Geometry: final body of the model. Coordinates: model frame, mm. Round coordinates to 2 decimals unless told otherwise and drop trailing zeros. Loops run counter-clockwise (first coordinate to the right, second up) from the corner with the lowest first, then second, coordinate; pieces in that order, holes last. Notation, with made-up numbers: (34, -17.75) - (93, -17.75) arc R25 ccw to (93, 1.25) - close; hole circle Ø4 at (12.5, -8). An arc over 180 degrees is marked (long way). Write item = value, one per line. Start each with the question number.
Item 1: Section D-D (y = 2.45). Count the separate pieces of the cut face and the enclosed holes in it, plus the area to 3 significant figures.
Item 2: Section C-C (x = -19). Return loops of the section in (y, z).
Item 3: Section A-A (x = 22). Return loops of the section in (y, z) (3 decimals), plus the area to 3 significant figures.
Item 4: Section B-B (z = -28). Return loops of the section in (x, y).
Item 5: Line query: line 1 (X direction, y = 1.5, z = -17.5); line 2 (Z direction, x = -22.5, y = 2.1); line 3 (X direction, y = 2.3, z = -9.5). Output: solid intervals per line, ascending. Write a range as from..to.
Item 6: First-contact query: pin 1 (1 mm diameter, centred on y = 1, z = -23.5, fed in from +X); pin 2 (2.5 mm diameter, centred on y = 2, z = -17.5, fed in from -X); pin 3 (2.5 mm diameter, centred on y = 2, z = -57.5, fed in from +X). Flat tips, straight axial feed; report the tip coordinate or a pass-through.
from build123d import *

# Parameters (mm, degrees)
SKETCH1_R           = 1.5875
SKETCH1_R_2         = 2.0955
SKETCH1_W           = 7.0612
SKETCH1_H           = 27.94
BOSS_EXTRUDE1_DEPTH = 4.699
FILLET1_R           = 2.54


with BuildPart() as part:
    # Sketch1 → Boss-Extrude1 (new body)
    with BuildSketch(Plane(origin=(0, 0, 0), x_dir=(1, 0, 0), z_dir=(0, 1, 0))):
        Polygon((0, 0), (30.48, 0), (30.48, 29.845), (32.385, 31.75), (32.385, 50.546), (-3.048, 50.546), (-3.048, 61.722), (-30.48, 61.722), (-30.48, 49.5427), (-35.2425, 44.7802), (-35.2425, 36.5252), (-30.48, 31.7627), (-30.48, 0), align=None)
        with Locations(Location((-0.9906, 40.6527, 0), (0, 0, 270))):
            Circle(SKETCH1_R, mode=Mode.SUBTRACT)
        with Locations(Location((-12.55014, 55.50916, 0), (0, 0, 270))):
            Circle(SKETCH1_R_2, mode=Mode.SUBTRACT)
        with Locations(Location((-22.40026, 55.50916, 0), (0, 0, 270))):
            Circle(SKETCH1_R_2, mode=Mode.SUBTRACT)
        with Locations(Location((-12.55014, 6.08584, 0), (0, 0, 270))):
            Circle(SKETCH1_R_2, mode=Mode.SUBTRACT)
        with Locations(Location((-22.40026, 6.08584, 0), (0, 0, 270))):
            Circle(SKETCH1_R_2, mode=Mode.SUBTRACT)
        Polygon((5.461, 5.715), (25.781, 5.715), (25.781, 38.0492), (28.575, 38.0492), (28.575, 46.736), (5.461, 46.736), (5.461, 43.2562), (2.5273, 43.2562), (2.5273, 38.0492), (5.461, 38.0492), align=None, mode=Mode.SUBTRACT)
        Polygon((-27.5082, 10.668), (-7.4422, 10.668), (-7.4422, 38.0492), (-4.5085, 38.0492), (-4.5085, 43.2562), (-7.4422, 43.2562), (-7.4422, 50.927), (-27.5082, 50.927), (-27.5082, 43.2562), (-32.5755, 43.2562), (-32.5755, 38.0492), (-27.5082, 38.0492), align=None, mode=Mode.SUBTRACT)
        with Locations((-0.9906, 20.32)):
            Rectangle(SKETCH1_W, SKETCH1_H, mode=Mode.SUBTRACT)
    extrude(amount=BOSS_EXTRUDE1_DEPTH)

    # Fillet1
    fillet1_edges = [part.edges().sort_by_distance(p)[0] for p in [
        (-3.048, 2.3495, -50.546),
        (32.385, 2.3495, -50.546),
        (32.385, 2.3495, -31.75),
        (30.48, 2.3495, -29.845),
        (30.48, 2.3495, 0),
        (-30.48, 2.3495, 0),
        (-30.48, 2.3495, -31.7627),
        (-35.2425, 2.3495, -36.5252),
        (-35.2425, 2.3495, -44.7802),
        (-30.48, 2.3495, -49.5427),
        (-30.48, 2.3495, -61.722),
        (-3.048, 2.3495, -61.722),
    ]]
    fillet(fillet1_edges, radius=FILLET1_R)


solid = part.part
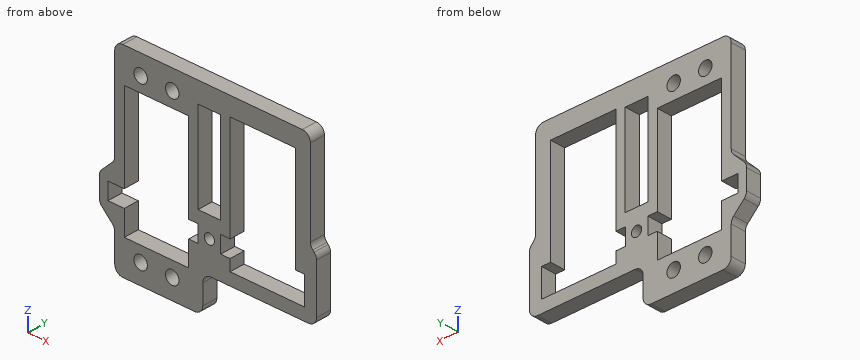
Taken from the geometry:
q1.separate_pieces = 1
q1.enclosed_holes = 8
q1.area = 1,500 mm^2
q2.outline = (0, -61.72) - (4.7, -61.72) - (4.7, -50.93) - (0, -50.93) - close; (0, -10.67) - (4.7, -10.67) - (4.7, 0) - (0, 0) - close
q3.outline = (0, -50.546) - (4.699, -50.546) - (4.699, -46.736) - (0, -46.736) - close; (0, -5.715) - (4.699, -5.715) - (4.699, 0) - (0, 0) - close
q3.area = 44.8 mm^2
q4.outline = (-30.48, 0) - (-27.51, 0) - (-27.51, 4.7) - (-30.48, 4.7) - close; (-7.44, 0) - (-4.52, 0) - (-4.52, 4.7) - (-7.44, 4.7) - close; (2.54, 0) - (5.46, 0) - (5.46, 4.7) - (2.54, 4.7) - close; (25.78, 0) - (30.48, 0) - (30.48, 4.7) - (25.78, 4.7) - close
q5.line_1 = -30.48..-27.51, -7.44..-4.52, 2.54..5.46, 25.78..30.48
q5.line_2 = -61.72..-57.6, -53.42..-50.93, -10.67..-8.18, -3.99..0
q5.line_3 = -30.48..-4.52, 2.54..5.46, 25.78..30.48
q6.pin_1 = 30.48
q6.pin_2 = -30.48
q6.pin_3 = -3.05
